Job drawing, mm, ordinate dimensions from the low corner. One solid piece. Round coordinates to 2 decimals unless told otherwise and drop trailing zeros. Loops run counter-clockwise (first coordinate to the right, second up) from the corner with the lowest first, then second, coordinate; pieces in that order, holes last. Notation, with made-up numbers: M 81,58.5 L 130,58.5 A34 cw 130,88.5 Z; hole C -24,30.5 d9. An arc over 180 degrees is marked long. One line per item, written item: value.
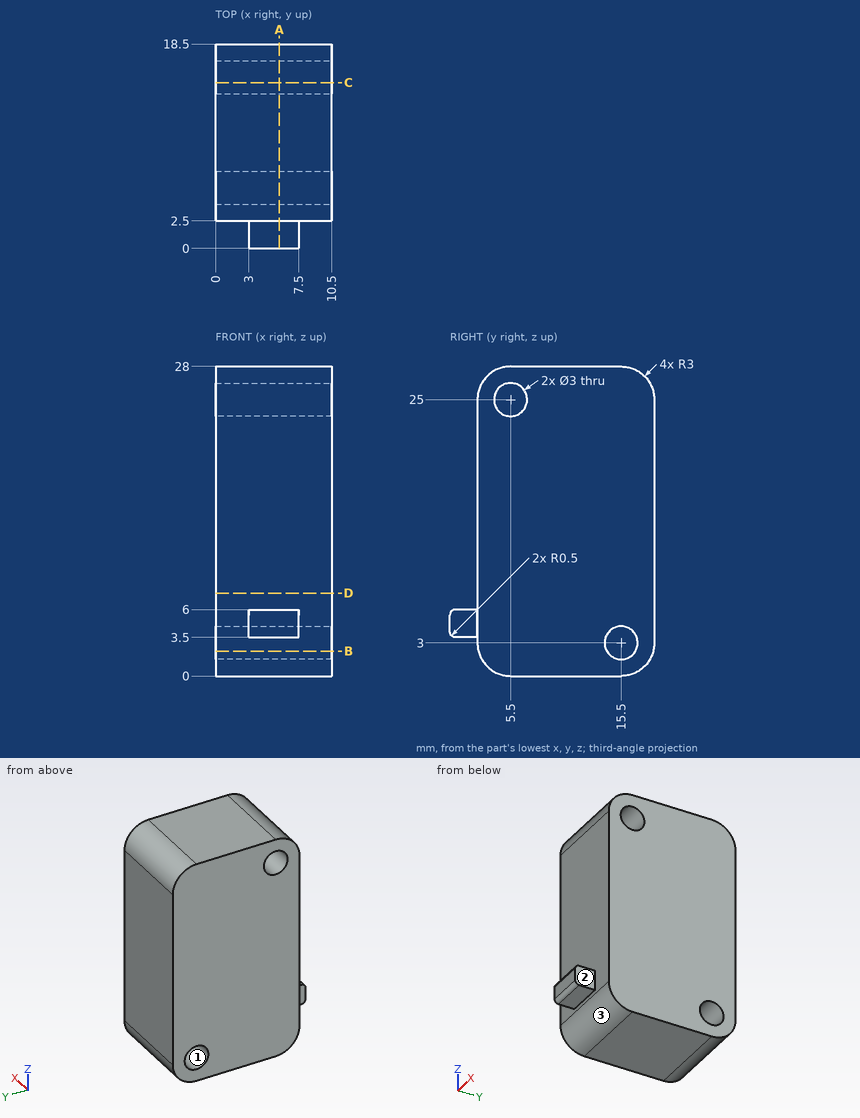
Item 1: Drop flat-ended pins along their axis: P1, Ø2.5, axis at y = 5.5, z = 25, coming from the -X side; P2, Ø1, axis at x = 5, y = 1.5, coming from the +Z side; P3, Ø1.5, axis at x = 5, y = 16.5, coming from the -Z side; P4, Ø5, axis at x = 4.5, z = 12, coming from the -Y side. Give the stop position or say it passes through.
Check values:
P1: passes through
P2: stops at z = 6
P3: stops at z = 0.01
P4: stops at y = 2.5
Item 2: Slice it at B-B, the plane z = 2.25. Give the cut face in (x, y).
Check values:
outline: M 0,2.6 L 10.5,2.6 L 10.5,14.2 L 0,14.2 Z; M 0,16.8 L 10.5,16.8 L 10.5,18.4 L 0,18.4 Z
Item 3: Slice it at D-D, the plane z = 7.5. Give the cut face in (x, y), and give its area (3 significant figures).
Check values:
outline: M 0,2.5 L 10.5,2.5 L 10.5,18.5 L 0,18.5 Z
area: 168 mm2
Item 4: Wall check: line 1 along Y through (x, z) = (7.75, 25); line 2 along Z through (x, y) = (7.25, 16.5); line 3 along Y through (x, z) = (9.5, 21.25). Give the ranges that are in metal, low to high.
Check values:
line 1: y = 2.5 to 4, 7 to 18.5
line 2: z = 0.17 to 1.88, 4.12 to 27.83
line 3: y = 2.5 to 18.5
Item 5: Slice it at C-C, the plane y = 15. Give the cut face in (x, z), and give its area (3 significant figures).
Check values:
outline: M 0,0 L 10.5,0 L 10.5,1.59 L 0,1.59 Z; M 0,4.41 L 10.5,4.41 L 10.5,28 L 0,28 Z
area: 264 mm2
Item 6: Slice it at A-A, the plane x = 5.75. Give the cut face in (y, z), and give its area (3 significant figures).
Check values:
outline: M 0,4 A0.5 ccw 0.5,3.5 L 2.5,3.5 L 2.5,3 A3 ccw 5.5,0 L 15.5,0 A3 ccw 18.5,3 L 18.5,25 A3 ccw 15.5,28 L 5.5,28 A3 ccw 2.5,25 L 2.5,6 L 0.5,6 A0.5 ccw 0,5.5 Z; hole C 5.5,25 d3; hole C 15.5,3 d3
area: 432 mm2
Item 7: Pull direction Y, two halves, no side cores. Call the marked faces 1, 2 and 3: pulls with the +Y half, pulls with the -Y half, needs draft (parallel to the pull), parting line crosses it, or undercut.
Check values:
face 1: undercut
face 2: needs draft
face 3: pulls with the -Y half
